The listing builds one solid part. Answer for the finished solid, in the listing's coordinates (mm). Face numbers are marked on the shaded views. A direction names the side the tool comes from. Round coordinates to 2 decimals unless told otherwise and drop trailing zeros. Write each loop counter-clockwise with the first axis right and the second up, starting at its lowest first coordinate (ties: lowest second). Pieces come first, ordered by that corner, then holes.
Item 1: Find section A-A on z = -4.75. Give the vertices of the cut face in (x, y), then the cut area to 3 significant figures.
Item 2: Find section C-C on y = 2.5. Give the vertices of the cut face in (x, z).
Item 3: For a pull along X with two mould halves and no side action, classify the marked faces 1, 2, 3 and 4 as +X half, -X half, draft (parallel to the pull), parting line (faces both ways), or undercut.
Item 4: Find section D-D on x = 6.25. Give the vertices of the cut face in (y, z).
Item 5: A tool of negligible diameter and unlimited length cuts with its end or side. For the marked faces 5, 6 and 7, from which of +Z, -Z, +X, -X, +Y, -Y can it reach the whole face along a straight path? Write none if from no direction.
Item 6: Find section B-B on x = 10.75. Give the vertices of the cut face in (y, z), then the cut area to 3 significant figures.
Item 7: Each of these flat-tipped pins is pushed along its axis until it touches: pin 1 (1.8 mm diameter, centred on x = 9.5, z = -4.5, fed in from -Y); pin 2 (2 mm diameter, centred on y = 4.5, z = -4, fed in from -X); pin 3 (6.5 mm diameter, centred on x = 5.5, z = -4.75, fed in from -Y). Where does it stop, or does it pass through?
Item 8: Find the intervals of material crossed by probe 1 along Z at (x, y) = (4.5, 13.5); probe 2 along X at (y, z) = (1.25, -4.75); probe 3 along Y at (x, z) = (4.5, -0.5), in increasing order.
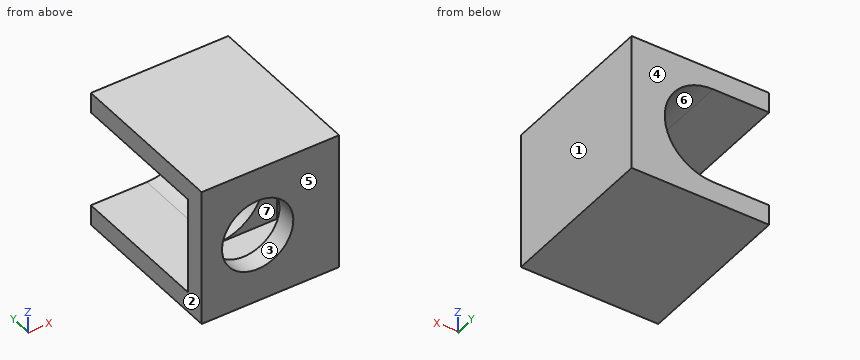
```python
from build123d import *

# Parameters (mm, degrees)
SKETCH_1_R          = 3.5
EXTRUDE_2_DEPTH     = 16
CUT_EXTRUDE_START   = 2
SKETCH_1_7_R        = 3.5
CUT_EXTRUDE_6_DEPTH = 4
SKETCH_1_9_R        = 3.5
CUT_EXTRUDE_8_DEPTH = 14


with BuildPart() as part:
    # Sketch 1 → Extrude 2 (new body)
    # profile 1 of 3: a face of its own
    with BuildSketch(Plane(origin=(0, 0, 0), x_dir=(1, 0, 0), z_dir=(0, 1, 0))):
        Polygon((0, 9.5), (0, 11.5), (5.5, 11.5), (13.5, 11.5), (13.5, -2), (5.5, -2), (0, -2), (0, 0), (5.5, 0), (11.5, 0), (11.5, 9.5), (5.5, 9.5), align=None)
    # profile 2 of 3: a face of its own
    with BuildSketch(Plane(origin=(0, 0, 0), x_dir=(1, 0, 0), z_dir=(0, 1, 0))):
        with BuildLine():
            Line((5.5, 9.5), (11.5, 9.5))
            Line((11.5, 9.5), (11.5, 0))
            Line((11.5, 0), (5.5, 0))
            ThreePointArc((5.5, 0), (10.25, 4.75), (5.5, 9.5))
        make_face()
    # profile 3 of 3: a face of its own
    with BuildSketch(Plane(origin=(0, 0, 0), x_dir=(1, 0, 0), z_dir=(0, 1, 0))):
        with BuildLine():
            ThreePointArc((5.5, 9.5), (10.25, 4.75), (5.5, 0))
            Line((5.5, 0), (0, 0))
            Line((0, 0), (0, 9.5))
            Line((0, 9.5), (5.5, 9.5))
        make_face()
        with Locations(Location((5.5, 4.75, 0), (0, 0, 270))):
            Circle(SKETCH_1_R, mode=Mode.SUBTRACT)
    extrude(amount=EXTRUDE_2_DEPTH)

    # Sketch 1_7 → Cut-Extrude 6 (cut)
    # profile 1 of 2: a face of its own
    with BuildSketch(Plane(origin=(0, 0, 0), x_dir=(1, 0, 0), z_dir=(0, 1, 0)).offset(CUT_EXTRUDE_START)):
        with BuildLine():
            ThreePointArc((5.5, 9.5), (10.25, 4.75), (5.5, 0))
            Line((5.5, 0), (0, 0))
            Line((0, 0), (0, 9.5))
            Line((0, 9.5), (5.5, 9.5))
        make_face()
        with Locations(Location((5.5, 4.75, 0), (0, 0, 270))):
            Circle(SKETCH_1_7_R, mode=Mode.SUBTRACT)
    # profile 2 of 2: a face of its own
    with BuildSketch(Plane(origin=(0, 0, 0), x_dir=(1, 0, 0), z_dir=(0, 1, 0)).offset(CUT_EXTRUDE_START)):
        with BuildLine():
            Line((5.5, 9.5), (11.5, 9.5))
            Line((11.5, 9.5), (11.5, 0))
            Line((11.5, 0), (5.5, 0))
            ThreePointArc((5.5, 0), (10.25, 4.75), (5.5, 9.5))
        make_face()
    extrude(amount=CUT_EXTRUDE_6_DEPTH, mode=Mode.SUBTRACT)

    # Sketch 1_9 → Cut-Extrude 8 (cut)
    with BuildSketch(Plane(origin=(0, 0, 0), x_dir=(1, 0, 0), z_dir=(0, 1, 0)).offset(CUT_EXTRUDE_START)):
        with BuildLine():
            ThreePointArc((5.5, 9.5), (10.25, 4.75), (5.5, 0))
            Line((5.5, 0), (0, 0))
            Line((0, 0), (0, 9.5))
            Line((0, 9.5), (5.5, 9.5))
        make_face()
        with Locations(Location((5.5, 4.75, 0), (0, 0, 270))):
            Circle(SKETCH_1_9_R, mode=Mode.SUBTRACT)
    extrude(amount=CUT_EXTRUDE_8_DEPTH, mode=Mode.SUBTRACT)


solid = part.part
```
Check values:
1. outline: (0, 0) - (2, 0) - (2, 2) - (0, 2) - close; (9, 0) - (13.5, 0) - (13.5, 16) - (10.25, 16) - (10.25, 6) - (11.5, 6) - (11.5, 2) - (9, 2) - close
1. area: 53.5 mm2
2. outline: (0, -11.5) - (13.5, -11.5) - (13.5, 2) - (0, 2) - (0, 0) - (11.5, 0) - (11.5, -9.5) - (0, -9.5) - close
3. face 1: +X half
3. face 2: -X half
3. face 3: undercut
3. face 4: draft
4. outline: (0, -11.5) - (16, -11.5) - (16, -9.44) - (6, -9.44) - (6, -9.5) - (2, -9.5) - (2, -8.17) - (0, -8.17) - close; (0, -1.33) - (2, -1.33) - (2, 0) - (6, 0) - (6, -0.06) - (16, -0.06) - (16, 2) - (0, 2) - close
5. face 5: +Z, -Z, +X, -X, -Y
5. face 6: -X, +Y
5. face 7: -X
6. outline: (0, -11.5) - (16, -11.5) - (16, 2) - (0, 2) - close; hole (2, -9.5) - (6, -9.5) - (6, 0) - (2, 0) - close
6. area: 178 mm2
7. pin 1: stops at y = 0
7. pin 2: stops at x = 11.5
7. pin 3: passes through
8. probe 1: z = -11.5 to -9.5, 0 to 2
8. probe 2: x = 0 to 2, 9 to 13.5
8. probe 3: y = 0 to 2
